Autodesk Inventor part; units mm, degrees
ref_plane "YZ Plane" through (0, 0, 0) normal (1, 0, 0) x (0, 1, 0)
ref_plane "XZ Plane" through (0, 0, 0) normal (0, 1, 0) x (-1, 0, 0)
ref_plane "XY Plane" through (0, 0, 0) normal (0, 0, 1) x (1, 0, 0)
sketch "Sketch1" plane through (0, 0, 0) normal (0, 0, 1) x (1, 0, 0)
  line L0 (0, 0) -> (28.575, 0)
  line L1 (28.575, 0) -> (28.575, 203.2)
  line L2 (28.575, 203.2) -> (0, 203.2)
  line L3 (0, 203.2) -> (0, 0)
  line L4 (31.75, 206.375) -> (31.75, 0)
  line L5 (-3.175, 0) -> (-3.175, 206.375)
  line L6 (-3.175, 206.375) -> (31.75, 206.375)
  line L7 (-3.175, 0) -> (31.75, 0)
  dimension "d0" = 28.575
  dimension "d1" = 203.2
  dimension "d2" = 3.175
  dimension "d24" = 3.175
  dimension "d25" = 3.175
extrude "Extrusion1" add sketch "Sketch1" along normal blind 28.575 contours L7 L5 L6 L4 L1 L2 L3
sketch "Sketch2" plane through (31.75, 0, 0) normal (1, 0, 0) x (0, 0, -1)
  line L0 (0, 0) -> (-28.575, 0)
  line L1 (0, 206.375) -> (0, 0)
  point P0 (-23.8125, 5.207)
  point P1 (-4.7625, 5.207)
  dimension "d5" = 5.207
  dimension "d6" = 19.05
  dimension "d7" = 28.575
  dimension "d8" = 4.7625
hole "Hole1" at (31.75, 5.207, 23.8125) at (31.75, 5.207, 4.7625) direction (-1, 0, 0) diameter 5.1054 end through all
sketch "Sketch3" plane through (-3.175, 206.375, 0) normal (0, 1, 0) x (1, 0, 0)
  line L0 (3.175, 0) -> (3.175, -28.575)
  line L1 (31.75, 0) -> (31.75, -28.575)
  point P0 (17.4625, -14.2875)
  point P1 (3.175, -14.2875)
  dimension "d16" = 14.2875
hole "Hole2" at (14.2875, 206.375, 14.2875) direction (0, -1, 0) diameter 6.7564 end through all
Input: part model. Units: mm. Frame: model coordinates. A direction names the side the tool comes from. Give positions to 0.01 mm unless a question says otherwise; leave off trailing zeros. Write each loop counter-clockwise with the first axis right and the second up, starting at its lowest first coordinate (ties: lowest second). Pieces come first, ordered by that corner, then holes. Notation, with made-up numbers: (-0.75, 74.25) -> (12.25, 74.25) arc R22 ccw to (12.25, 92.25) -> close; hole circle Ø4 at (80.5, 76). An arc over 180 degrees is marked (long way). Use one line per item in the form item = value. Start each with the question number.
1) Section query C-C on z = 24.5. Return the cut outline in (x, y) (3 decimals), then the cut area to 3 significant figures.
2) Draft query along X for faces 3 (the flat face through (18, 203.2, 14)), 4 (the cylindrical face through (30.14, 6.185, 21.454)), 5 (the cylindrical face through (15.6, 204.8, 17.4)), 6 (the flat face through (31.75, 105, 14)). Return one class per face: pulls with the +X half, pulls with the -X half, needs draft (parallel to the pull), parting line crosses it, or undercut.
3) Pin query (flat end, axial travel): pin 1 (3 mm diameter, centred on x = 18, z = 16, fed in from -Y). Return the tip coordinate at first contact, or that it passes through.
4) Section query D-D on x = 7. Return the cut outline in (y, z) (3 decimals).
5) Ray query, probe 1 along X at (y, z) = (82, 10.75) (3 decimals); probe 2 along Y at (x, z) = (6.5, 12) (3 decimals). Return the intervals inside material, ascending. Write a range as from..to.
6) Set-up query: faces 1 (the flat face through (-3.175, 102, 14)), 2 (the flat face through (0, 103, 14)). Return all of +Z, -Z, +X, -X, +Y, -Y with unobstructed straight access to the full face (end or side cutting, diameter ignored); none if empty.
7) Section query B-B on z = 13.75. Return the cut outline in (x, y) (3 decimals), then the cut area to 3 significant figures.
8) Section query A-A on y = 43. Return the cut outline in (x, z) (3 decimals), then the cut area to 3 significant figures.
Outcome:
q1.outline = (-3.175, 0) -> (0, 0) -> (0, 2.749) -> (-3.175, 2.749) -> close; (-3.175, 7.665) -> (0, 7.665) -> (0, 203.2) -> (28.575, 203.2) -> (28.575, 7.665) -> (31.75, 7.665) -> (31.75, 206.375) -> (-3.175, 206.375) -> close; (28.575, 0) -> (31.75, 0) -> (31.75, 2.749) -> (28.575, 2.749) -> close
q1.area = 1,370 mm^2
q2.face_3 = undercut
q2.face_4 = needs draft
q2.face_5 = undercut
q2.face_6 = pulls with the +X half
q3.pin_1 = 203.2
q4.outline = (203.2, 0) -> (206.375, 0) -> (206.375, 28.575) -> (203.2, 28.575) -> close
q5.probe_1 = -3.175..0, 28.575..31.75
q5.probe_2 = 203.2..206.375
q6.face_1 = +Z, -Z, -X, +Y, -Y
q6.face_2 = +Z, -Z, -Y
q7.outline = (-3.175, 0) -> (0, 0) -> (0, 203.2) -> (10.952, 203.2) -> (10.952, 206.375) -> (-3.175, 206.375) -> close; (17.623, 203.2) -> (28.575, 203.2) -> (28.575, 0) -> (31.75, 0) -> (31.75, 206.375) -> (17.623, 206.375) -> close
q7.area = 1,380 mm^2
q8.outline = (-3.175, 0) -> (0, 0) -> (0, 28.575) -> (-3.175, 28.575) -> close; (28.575, 0) -> (31.75, 0) -> (31.75, 28.575) -> (28.575, 28.575) -> close
q8.area = 181 mm^2
